Can you work these out from the model? Positions are in its coordinate system, mm. A direction names the side the tool comes from. Coordinates: 2 decimals unless noted, no trailing zeros. Order: outer loops, then holes, each group sorted by start corner. A loop starts at its lowest first (then second) coordinate and runs counter-clockwise, first axis right, second up.
Autodesk Inventor part; units mm, degrees
ref_plane "YZ Plane" through (0, 0, 0) normal (1, 0, 0) x (0, 1, 0)
ref_plane "XZ Plane" through (0, 0, 0) normal (0, 1, 0) x (-1, 0, 0)
ref_plane "XY Plane" through (0, 0, 0) normal (0, 0, 1) x (1, 0, 0)
sketch "Sketch1" plane through (0, 0, 0) normal (0, 1, 0) x (-1, 0, 0)
  line L0 (-0.15, 0.475) -> (0.15, 0.475)
  line L1 (0.15, 0.475) -> (0.15, -0.475)
  line L2 (0.15, -0.475) -> (-0.15, -0.475)
  line L3 (-0.15, -0.475) -> (-0.15, 0.475)
  line L4 (-0.15, 0.475) -> (0.15, -0.475) construction
  line L5 (0.15, 0.475) -> (-0.15, -0.475) construction
  line L6 (-0.15, 5.475) -> (0.15, 5.475)
  line L7 (0.15, 5.475) -> (0.15, 4.525)
  line L8 (0.15, 4.525) -> (-0.15, 4.525)
  line L9 (-0.15, 4.525) -> (-0.15, 5.475)
  line L10 (-0.15, 5.475) -> (0.15, 4.525) construction
  line L11 (0.15, 5.475) -> (-0.15, 4.525) construction
  line L12 (0, -1.665) -> (0, 6.665) construction
  line L13 (-14.61, 0) -> (2.61, 0) construction
  line L14 (-12.15, 0.475) -> (-11.85, 0.475)
  line L15 (-11.85, 0.475) -> (-11.85, -0.475)
  line L16 (-11.85, -0.475) -> (-12.15, -0.475)
  line L17 (-12.15, -0.475) -> (-12.15, 0.475)
  line L18 (-12.15, 0.475) -> (-11.85, -0.475) construction
  line L19 (-11.85, 0.475) -> (-12.15, -0.475) construction
  line L20 (-12.15, 5.475) -> (-11.85, 5.475)
  line L21 (-11.85, 5.475) -> (-11.85, 4.525)
  line L22 (-11.85, 4.525) -> (-12.15, 4.525)
  line L23 (-12.15, 4.525) -> (-12.15, 5.475)
  line L24 (-12.15, 5.475) -> (-11.85, 4.525) construction
  line L25 (-11.85, 5.475) -> (-12.15, 4.525) construction
  line L26 (-12, 0) -> (-12, 5) construction
  line L27 (-12, 5) -> (0, 5) construction
  point P0 (0, 0)
  point P1 (0, 5)
  point P2 (-12, 0)
  dimension "d0" = 0.95
  dimension "d1" = 0.3
  dimension "d2" = 0.95
  dimension "d3" = 0.3
  dimension "d4" = 5
  dimension "d5" = 0.95
  dimension "d6" = 0.3
  dimension "d7" = 12
  dimension "d8" = 0.95
  dimension "d9" = 0.3
extrude "Extrusion1" add sketch "Sketch1" against normal blind 3
sketch "Sketch2" plane through (0, 0, 0) normal (0, 1, 0) x (-1, 0, 0)
  line L0 (0, -3.5) -> (-12, -3.5)
  line L1 (-12, -3.5) -> (-12, 8.5)
  line L2 (-12, 8.5) -> (0, 8.5)
  line L3 (0, 8.5) -> (0, -3.5)
  line L4 (0, -3.5) -> (-12, 8.5) construction
  line L5 (0, 8.5) -> (-12, -3.5) construction
  line L6 (-12.15, 5.475) -> (-11.85, 5.475) construction
  line L7 (-12.15, 4.525) -> (-12.15, 5.475) construction
  line L8 (-11.85, 4.525) -> (-12.15, 4.525) construction
  line L9 (-11.85, 5.475) -> (-11.85, 4.525) construction
  line L10 (-11.85, 5.475) -> (-11.85, 4.525) construction
  line L11 (-11.85, 5) -> (-12.15, 5) construction
  point P0 (0, 0)
  point P1 (-6, 2.5)
  point P2 (-6, 2.5)
  dimension "d12" = 12
  dimension "d13" = 12
  dimension "d14" = 6
  dimension "d15" = 2.5
extrude "Extrusion2" add sketch "Sketch2" along normal blind 2.5
sketch "Sketch3" plane through (0, 2.5, 0) normal (0, 1, 0) x (1, 0, 0)
  line L0 (12, 3.5) -> (0, 3.5) construction
  line L1 (0, 3.5) -> (0, -8.5) construction
  line L2 (0, -8.5) -> (12, -8.5) construction
  line L3 (12, -8.5) -> (12, 3.5) construction
  line L4 (0, 3.5) -> (12, 3.5) construction
  line L5 (0, 3.5) -> (12, -8.5) construction
  line L6 (12, -8.5) -> (0, -8.5) construction
  line L7 (0, -8.5) -> (12, 3.5) construction
  circle A0 centre (6, -2.5) radius 3.35
  point P0 (0, 0)
  dimension "d18" = 6.7
extrude "Extrusion3" add sketch "Sketch3" along normal blind 1
sketch "Sketch4" plane through (6, 3.5, 2.5) normal (0, 1, 0) x (1, 0, 0)
  circle A0 centre (0, 0) radius 3.35
  line L0 (-3, -3) -> (3, -3)
  line L1 (3, -3) -> (3, 3)
  line L2 (3, 3) -> (-3, 3)
  line L3 (-3, 3) -> (-3, -3)
  line L4 (-3, -3) -> (3, 3) construction
  line L5 (3, -3) -> (-3, 3) construction
  point P0 (-6, 2.5)
  dimension "d21" = 6
  dimension "d22" = 6
extrude "Extrusion4" add sketch "Sketch4" along normal blind 1.2 contours L1 A0 L0 L3 L2 | A0 L2 L1 | L1 L0 A0 | A0 L3 L2 | L0 L3 A0
sketch "Sketch5" plane through (6, 4.7, 2.5) normal (0, 1, 0) x (1, 0, 0)
  circle A0 centre (0, 0) radius 3.35 construction
  line L0 (6, 6) -> (-6, 6) construction
  line L1 (-6, 6) -> (-6, -6) construction
  line L2 (-6, -6) -> (6, -6) construction
  line L3 (6, -6) -> (6, 6) construction
  line L4 (-4.575, -4.575) -> (4.575, -4.575)
  line L5 (4.575, -4.575) -> (4.575, 4.575)
  line L6 (4.575, 4.575) -> (-4.575, 4.575)
  line L7 (-4.575, 4.575) -> (-4.575, -4.575)
  line L8 (-4.575, -4.575) -> (4.575, 4.575) construction
  line L9 (4.575, -4.575) -> (-4.575, 4.575) construction
  point P0 (-6, 2.5)
  dimension "d25" = 9.15
  dimension "d26" = 9.15
extrude "Extrusion5" add sketch "Sketch5" along normal blind 5.5
equation "\"d13\" = d12"
equation "\"d22\" = d21"
equation "\"d26\" = d25"
properties part number "NINIGI_TACTS-24N"
1. Imagine slicing it at B-B on z = 3. Please give me the cut outline in (x, y) (3 decimals), then the cut area to 4 significant figures.
Completed:
outline: (0, 0) - (12, 0) - (12, 2.5) - (9.312, 2.5) - (9.312, 3.5) - (9, 3.5) - (9, 4.7) - (10.575, 4.7) - (10.575, 10.2) - (1.425, 10.2) - (1.425, 4.7) - (3, 4.7) - (3, 3.5) - (2.688, 3.5) - (2.688, 2.5) - (0, 2.5) - close
area: 94.15 mm2
2. Imagine slicing it at A-A on x = 9.75. Please give me the cut outline in (y, z) (3 decimals).
Completed:
outline: (0, -3.5) - (2.5, -3.5) - (2.5, 8.5) - (0, 8.5) - close; (4.7, -2.075) - (10.2, -2.075) - (10.2, 7.075) - (4.7, 7.075) - close
3. Imagine slicing it at D-D on y = 8. Please give me the cut outline in (x, z) (3 decimals), then the cut area to 3 significant figures.
Completed:
outline: (1.425, -2.075) - (10.575, -2.075) - (10.575, 7.075) - (1.425, 7.075) - close
area: 83.7 mm2
4. Please list where these lines run through material, in increasing order: probe 1 along X at (y, z) = (-0.25, -0.25); probe 2 along Y at (x, z) = (6, -1.5); probe 3 along Y at (x, z) = (10.75, 8.25).
Completed:
probe 1: x = -0.15 to 0.15, 11.85 to 12.15
probe 2: y = 0 to 2.5, 4.7 to 10.2
probe 3: y = 0 to 2.5
5. Imagine slicing it at C-C on x = 6. Please give me the cut outline in (y, z) (3 decimals), then the cut area to 3 significant figures.
Completed:
outline: (0, -3.5) - (2.5, -3.5) - (2.5, -0.85) - (3.5, -0.85) - (3.5, -0.5) - (4.7, -0.5) - (4.7, -2.075) - (10.2, -2.075) - (10.2, 7.075) - (4.7, 7.075) - (4.7, 5.5) - (3.5, 5.5) - (3.5, 5.85) - (2.5, 5.85) - (2.5, 8.5) - (0, 8.5) - close
area: 94.2 mm2
6. I'm going to push flat-ended pins straight in: pin 1 (0.5 mm diameter, centred on x = 8, z = 0, fed in from -Y); pin 2 (6 mm diameter, centred on y = 5, z = -1, fed in from -X); pin 3 (1 mm diameter, centred on x = 2, y = -1, fed in from +Z). Where does each tip first touch, or does it pass through?
Completed:
pin 1: stops at y = 0
pin 2: stops at x = 0
pin 3: passes through
7. Thinking about a two-plate mould opening in Y: for faces 1 (the flat face through (-0.15, -1, 5)), 2 (the flat face through (6, 10.2, 2)), 3 (the flat face through (8.6, 3.5, -0.1)), which applies, pulls with the +Y half, pulls with the -Y half, needs draft (parallel to the pull), parting line crosses it, or undercut?
Completed:
face 1: needs draft
face 2: pulls with the +Y half
face 3: undercut
8. On a 3-axis mill with a long thin cutter (end or side, diameter ignored), from which of +Z, -Z, +X, -X, +Y, -Y can I reach the whole of each face in a straight line? I mean faces 4 (the flat face through (3.4, 3.5, 5.1)), 5 (the flat face through (6, 7, 7.075)), 6 (the flat face through (3.4, 3.5, -0.1)), 7 (the flat face through (11.85, -1, 5)), 8 (the cylindrical face through (7.55, 2.99, -0.47)). Say none if no direction works.
Completed:
face 4: +Z, -X
face 5: +Z, +X, -X, +Y
face 6: -Z, -X
face 7: +Z, -Z, -Y
face 8: none
